Could you check a few things on this model? Use its own coordinates, in mm. Face numbers are marked on the shaded views. A direction names the side the tool comes from. Round coordinates to 2 decimals unless told otherwise and drop trailing zeros. Write each loop counter-clockwise with the first axis right and the second up, starting at its lowest first coordinate (ties: lowest second). Pieces come first, ordered by that corner, then holes. Notation, with made-up numbers: (42, 9) -> (79, 9) arc R34 ccw to (79, 48) -> close; hole circle Ø2 at (-19.5, -27.5). An arc over 180 degrees is marked (long way). Answer as CSV lines item,"result". Start each with the question number.
Q1. Imagine slicing it at A-A on y = 9. Please give me the cut outline in (x, z), and give its area (3 significant figures).
Q2. If I drill on line 1 (Y direction, x = 13.25, z = 0.95); line 2 (Z direction, x = 0, y = -33.3); line 3 (X direction, y = -17.5, z = 23), over which ranges is the centre line in solid material (lowest first)? Write a range as [from, to].
Q3. Imagine slicing it at D-D on y = -23.5. Please give me the cut outline in (x, z).
Q4. For the marked faces 4 and 5, which set-ups out of +Z, -Z, +X, -X, +Y, -Y let a thin tool reach every point of the face, with its end or its side?
Q5. Imagine slicing it at C-C on x = 13.25. Give the number of separate pieces and of enclosed holes in the cut face, and give its area (3 significant figures).
Q6. If we mould it in two halves opening along X, with no side actions, what happens to the marked faces 1, 2 and 3? For each: pulls with the +X half, pulls with the -X half, needs draft (parallel to the pull), parting line crosses it, or undercut.
Q7. Will these pins go through, and if not, where does the flat tip stop? pin 1 Ø2.5 at (y, z) = (13, 25) entering from -X; pin 2 Ø1 at (x, z) = (-11.5, 22) entering from -Y; pin 3 Ø2 at (x, z) = (-20, 25) entering from +Y; pin 4 Ø1.6 at (x, z) = (-20.5, 25) entering from -Y.
Q8. Imagine slicing it at B-B on y = -31.5. Please give me the cut outline in (x, z), and give its area (3 significant figures).
from build123d import *

# Parameters (mm, degrees)
F4_DEPTH     = 23
F5_DEPTH     = 2
F6_R         = 11.5
F6_R_2       = 10.5
F7_DEPTH     = 6
F8_DEPTH     = 25
F9_T4_ANGLE  = 179.9999999711
F9_T10_ANGLE = 89.9999998967
F9_T15_ANGLE = 90.0000001322
F10_R        = 1.5
F11_DEPTH    = 2.001
F12_W        = 1.9858112633
F12_H        = 10
F13_DEPTH    = 5
F14_R        = 2
F15_W        = 6
F15_H        = 2
F16_DEPTH    = 42.001


# Not quite as in the source:
# - a fillet or chamfer that OpenCascade refuses, or shapes differently, is made with other operations: its cross-section is extruded or revolved along the edge and cut away or added


with BuildPart() as f4:
    # F3 (on Top) → F4 (new body)
    with BuildSketch(Plane.XY):
        with BuildLine():
            Line((18, 30), (-18, 30))
            ThreePointArc((-18, 30), (-20.1213203436, 29.1213203436), (-21, 27))
            Line((-21, 27), (-21, -27))
            ThreePointArc((-21, -27), (-20.1213203436, -29.1213203436), (-18, -30))
            Line((-18, -30), (18, -30))
            ThreePointArc((18, -30), (20.1213203436, -29.1213203436), (21, -27))
            Line((21, -27), (21, 27))
            ThreePointArc((21, 27), (20.1213203436, 29.1213203436), (18, 30))
        make_face()
        with BuildLine():
            ThreePointArc((-19, 25), (-18.1213203436, 27.1213203436), (-16, 28))
            Line((-16, 28), (16, 28))
            ThreePointArc((16, 28), (18.1213203436, 27.1213203436), (19, 25))
            Line((19, 25), (19, -25))
            ThreePointArc((19, -25), (18.1213203436, -27.1213203436), (16, -28))
            Line((16, -28), (-16, -28))
            ThreePointArc((-16, -28), (-18.1213203436, -27.1213203436), (-19, -25))
            Line((-19, -25), (-19, 25))
        make_face(mode=Mode.SUBTRACT)
    extrude(amount=F4_DEPTH)

    # F3 (on Top) → F5 (join)
    with BuildSketch(Plane.XY):
        with BuildLine():
            Line((16, 28), (-16, 28))
            ThreePointArc((-16, 28), (-18.1213203436, 27.1213203436), (-19, 25))
            Line((-19, 25), (-19, -25))
            ThreePointArc((-19, -25), (-18.1213203436, -27.1213203436), (-16, -28))
            Line((-16, -28), (16, -28))
            ThreePointArc((16, -28), (18.1213203436, -27.1213203436), (19, -25))
            Line((19, -25), (19, 25))
            ThreePointArc((19, 25), (18.1213203436, 27.1213203436), (16, 28))
        make_face()
    extrude(amount=F5_DEPTH)

    # F6 (on face) → F7 (join)
    with BuildSketch(Plane.XZ.offset(30)):
        with Locations((0, 11.5)):
            Circle(F6_R)
        with Locations((0, 11.5)):
            Circle(F6_R_2, mode=Mode.SUBTRACT)
    extrude(amount=F7_DEPTH)

    # F8 (cut): a face of the model
    f8_faces = [f4.faces().sort_by_distance(p)[0] for p in [
        (0, -30, 11.5),
    ]]
    extrude(f8_faces, amount=-F8_DEPTH, mode=Mode.SUBTRACT)

    # F9: chamfer of 5 on 1 edges, made by hand


with BuildPart() as f9_tool2:
    # F9_s3 → F9_t4 (revolve)
    with BuildSketch(Plane.YZ):
        Polygon((-30, 28), (-35, 23), (-30, 23), align=None)
    revolve(axis=Axis((0, -30, 11.5), (0, -1, 0)), revolution_arc=F9_T4_ANGLE)

    split(bisect_by=Plane.XY, keep=Keep.TOP)

    split(bisect_by=Plane.XY.offset(23), keep=Keep.BOTTOM)


with BuildPart() as f4_1:
    add(f4.part)

    # F9_t1: union F9_tool2
    add(f9_tool2.part)


with BuildPart() as f9_tool8:
    # F9_s9 → F9_t10 (revolve)
    with BuildSketch(Plane.XY.offset(11.5)):
        Polygon((16.5, -30), (11.5, -35), (11.5, -30), align=None)
    revolve(axis=Axis((0, -30, 11.5), (0, -1, 0)), revolution_arc=F9_T10_ANGLE)

    split(bisect_by=Plane.XY.offset(23), keep=Keep.BOTTOM)


with BuildPart() as f4_2:
    add(f4_1.part)

    # F9_t7: union F9_tool8
    add(f9_tool8.part)


with BuildPart() as f9_tool13:
    # F9_s14 → F9_t15 (revolve)
    with BuildSketch(Plane.YZ):
        Polygon((-30, -5), (-35, 0), (-30, 0), align=None)
    revolve(axis=Axis((0, -30, 11.5), (0, -1, 0)), revolution_arc=F9_T15_ANGLE)

    split(bisect_by=Plane.XY, keep=Keep.TOP)


with BuildPart() as f4_3:
    add(f4_2.part)

    # F9_t12: union F9_tool13
    add(f9_tool13.part)

    # F10 (on face) → F11 (cut, through all)
    with BuildSketch(Plane.XY.offset(2)):
        with Locations((-13.25, 18)):
            Circle(F10_R)
        with Locations((-13.25, -18)):
            Circle(F10_R)
        with Locations((13.25, 18)):
            Circle(F10_R)
        with Locations((13.25, -18)):
            Circle(F10_R)
    extrude(amount=-F11_DEPTH, mode=Mode.SUBTRACT)

    # F12 (on face) → F13 (join)
    with BuildSketch(Plane.XY.offset(23)):
        with Locations((-20.0070943683, 15)):
            Rectangle(F12_W, F12_H)
        with Locations((-20.0070943683, -15)):
            Rectangle(F12_W, F12_H)
        with Locations((20.0070943683, 15)):
            Rectangle(F12_W, F12_H)
        with Locations((20.0070943683, -15)):
            Rectangle(F12_W, F12_H)
    extrude(amount=F13_DEPTH)

    # F14
    f14_edges = [f4_3.edges().sort_by_distance(p)[0] for p in [
        (-20.007094, -20, 28),
        (-20.007094, -10, 28),
        (-20.007094, 10, 28),
        (-20.007094, 20, 28),
        (20.007094, 20, 28),
        (20.007094, 10, 28),
        (20.007094, -10, 28),
        (20.007094, -20, 28),
    ]]
    fillet(f14_edges, radius=F14_R)

    # F15 (on face) → F16 (cut, through all)
    with BuildSketch(Plane(origin=(-21, 0, 0), x_dir=(0, -1, 0), z_dir=(-1, 0, 0))):
        with Locations((-15, 25)):
            Rectangle(F15_W, F15_H)
        with Locations((15, 25)):
            Rectangle(F15_W, F15_H)
    extrude(amount=-F16_DEPTH, mode=Mode.SUBTRACT)


solid = f4_3.part
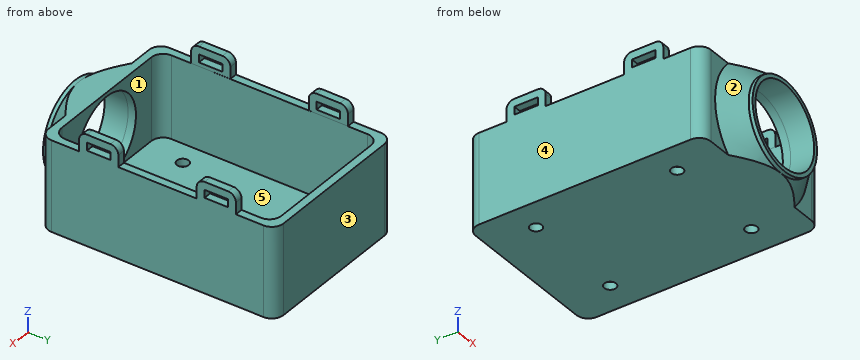
Checks:
1,outline,"(-21, 0) -> (21, 0) -> (21, 23) -> (19, 23) -> (19, 2) -> (-19, 2) -> (-19, 23) -> (-21, 23) -> close"
1,area,"168 mm^2"
2,line 1,"[-30, -19.5], [-16.5, 16.5], [19.5, 30]"
2,line 2,"[0, 1], [22, 23]"
2,line 3,"[-21, -19.01], [19.01, 21]"
3,outline,"(-21, 0) -> (21, 0) -> (21, 23) -> (19, 23) -> (19, 2) -> (4.47, 2) arc R10.5 cw to (-4.47, 2) -> (-19, 2) -> (-19, 23) -> (-21, 23) -> close"
4,face 4,"+Z, -Z, -X, +Y, -Y"
4,face 5,"+Z"
5,separate pieces,"3"
5,enclosed holes,"0"
5,area,"234 mm^2"
6,face 1,"undercut"
6,face 2,"pulls with the -X half"
6,face 3,"needs draft"
7,pin 1,"x = -21"
7,pin 2,"y = -31.43"
7,pin 3,"y = 20"
7,pin 4,"y = -20"
8,outline,"(-9.63, 0) -> (9.63, 0) arc R15 ccw to (9.63, 23) -> (-9.63, 23) arc R15 ccw to start; hole circle Ø21 at (0, 11.5)"
8,area,"268 mm^2"
